Autodesk Inventor part; units mm, degrees
ref_plane "YZ Plane" through (0, 0, 0) normal (1, 0, 0) x (0, 1, 0)
ref_plane "XZ Plane" through (0, 0, 0) normal (0, 1, 0) x (-1, 0, 0)
ref_plane "XY Plane" through (0, 0, 0) normal (0, 0, 1) x (1, 0, 0)
sketch "Skizze1" plane through (0, 0, 0) normal (0, 0, 1) x (1, 0, 0)
  circle A0 centre (0, 0) radius 8
  line L0 (-5.5, 0) -> (5.5, 0) construction
  circle A1 centre (0, 0) radius 3
  circle A2 centre (0, 0) radius 1.5
  arc A3 (-1.118, 1) -> (1.118, 1) centre (0, 0) ccw construction
  line L1 (-1.118, 1) -> (1.118, 1)
  dimension "d3" = 3
  dimension "d0" = 16
  dimension "d1" = 11
  dimension "d2" = 6
  dimension "d4" = 2.5
extrude "Extrusion1" add sketch "Skizze1" along normal blind 2 contours A1 | A2 L1 | L1 A2
sketch "Skizze2" plane through (0, 0, 2) normal (0, 0, 1) x (1, 0, 0)
  circle A0 centre (0, 0) radius 1.5
extrude "Extrusion2" add sketch "Skizze2" along normal blind 1
sketch "Skizze3" plane through (0, 0, 3) normal (0, 0, 1) x (1, 0, 0)
  circle A0 centre (0, 0) radius 1.5
  line L0 (-1.118, 1) -> (1.118, 1)
  circle A1 centre (0, 0) radius 1.5
extrude "Extrusion3" add sketch "Skizze3" along normal blind 7 contours A0 L0 picked at (0.0594, 0.1702)
extrude "Extrusion4" add sketch "Skizze1" against normal blind 14.5 contours A0 | A1 | A2 L1 | L1 A2
sketch "Skizze4" plane through (0, 0, -14.5) normal (0, 0, -1) x (-1, 0, 0)
  circle A0 centre (0, 0) radius 8
  arc A1 (-4.5983, 5.925) -> (-4.5983, -5.925) centre (0, 0) ccw
  arc A2 (4.5983, -5.925) -> (4.5983, 5.925) centre (0, 0) ccw
  line L0 (-4.5983, 5.925) -> (4.5983, 5.925)
  line L1 (4.5983, -5.925) -> (-4.5983, -5.925)
  dimension "d14" = 7.5
  dimension "d15" = 11.85
extrude "Extrusion5" add sketch "Skizze4" along normal blind 30 contours L0 A2 L1 A1
hole "Bohrung1" at (-5.5, 0, 0) at (5.5, 0, 0) direction (0, 0, -1) diameter 1.567 depth 3 tip angle 118
properties part number "dc-motor_12V_60U-min" material "Aluminium 6061"
For this review, take the finished solid that the model builds, in its own axes (mm). A direction names the side the tool comes from. Coordinates: 2 decimals unless noted, no trailing zeros. Write each loop counter-clockwise with the first axis right and the second up, starting at its lowest first coordinate (ties: lowest second). Pieces come first, ordered by that corner, then holes. Notation, with made-up numbers: (16, 50.5) - (64, 50.5) arc R33 cw to (64, 87.5) - close; hole circle Ø1 at (38, 69). An arc over 180 degrees is marked (long way). Answer in a Markdown table with one row per item. Add a question column.
Q1. For probe 1 along Z at (x, y) = (6.25, 4.5); probe 2 along Z at (x, y) = (-1.75, -3); probe 3 along Y at (x, z) = (-5.5, -0.85), list the stretches that pass through material, from the lowest coordinate up.
Q2. We need section D-D, the plane y = -6.75. State the section outline as (x, z) points, and give its area (3 significant figures).
Q3. Tool access review of faces 4 (the flat face through (0, -5.925, -29)), 5 (the flat face through (0, 7, -14.5)), 6 (the flat face through (0, 1, 6)), 7 (the flat face through (3.4, 0.1, 0)): name each direction out of +Z, -Z, +X, -X, +Y, -Y from which nothing blocks a thin tool from reaching the whole face with its end or side.
Q4. We need section C-C, the plane z = -32. State the section outline as (x, y) points (3 decimals).
Q5. We need section A-A, the plane x = -0.5. State the section outline as (y, z) points (3 decimals), and give its area (3 significant figures).
Q6. Draft analysis for pull direction Y (two halves, no side actions). For faces 1 (the flat face through (1.3, -1.3, 2)), 2 (the cylindrical face through (-6.277, 0.102, -1.521)), 3 (the cylindrical face through (-7.5, 0.1, -29.3)), state which applies: +Y half, -Y half, draft (parallel to the pull), parting line (faces both ways), or undercut.
Q7. For P1, Ø1.5, axis at y = -0.5, z = 2.5, coming from the +X side; P2, Ø2, axis at x = 5.5, y = 3, coming from the +Z side; P3, Ø0.6, axis at x = -0.5, y = 1.5, coming from the +Z side, all flat-tipped, find the tip position at first contact; note any pin that passes through.
Q8. We need section B-B, the plane y = 2. State the section outline as (x, z) points.
Answer list:
| question | item | result |
|---|---|---|
| 1 | probe 1 | z = -14.5 to 0 |
| 1 | probe 2 | z = -44.5 to 0 |
| 1 | probe 3 | y = -5.81 to -0.78, 0.78 to 5.81 |
| 2 | outline | (-4.29, -14.5) - (4.29, -14.5) - (4.29, 0) - (-4.29, 0) - close |
| 2 | area | 125 mm2 |
| 3 | face 4 | -Z, +X, -X, -Y |
| 3 | face 5 | -Z |
| 3 | face 6 | +Z, +X, -X, +Y |
| 3 | face 7 | +Z |
| 4 | outline | (-4.598, -5.925) - (4.598, -5.925) arc R7.5 ccw to (4.598, 5.925) - (-4.598, 5.925) arc R7.5 ccw to start |
| 5 | outline | (-7.984, -14.5) - (-5.925, -14.5) - (-5.925, -44.5) - (5.925, -44.5) - (5.925, -14.5) - (7.984, -14.5) - (7.984, 0) - (2.958, 0) - (2.958, 2) - (1.414, 2) - (1.414, 3) - (1, 3) - (1, 10) - (-1.414, 10) - (-1.414, 2) - (-2.958, 2) - (-2.958, 0) - (-7.984, 0) - close |
| 5 | area | 619 mm2 |
| 6 | face 1 | draft |
| 6 | face 2 | undercut |
| 6 | face 3 | parting line |
| 7 | P1 | stops at x = 3 |
| 7 | P2 | stops at z = 0 |
| 7 | P3 | stops at z = 3 |
| 8 | outline | (-7.75, -14.5) - (-7.23, -14.5) - (-7.23, -44.5) - (7.23, -44.5) - (7.23, -14.5) - (7.75, -14.5) - (7.75, 0) - (2.24, 0) - (2.24, 2) - (-2.24, 2) - (-2.24, 0) - (-7.75, 0) - close |
